Geometry check sheet. Reference: the model listing, model coordinates, mm. A direction names the side the tool comes from. Coordinates: 2 decimals unless noted, no trailing zeros. Order: outer loops, then holes, each group sorted by start corner. A loop starts at its lowest first (then second) coordinate and runs counter-clockwise, first axis right, second up.
```python
from build123d import *

# Parameters (mm, degrees)
SKETCH1_W     = 3.175
SKETCH1_H     = 12.7
CHAMFER1_SIZE = 1.27


with BuildPart() as part:
    # Sketch1 → Revolve1 (revolve)
    with BuildSketch(Plane.XY, mode=Mode.PRIVATE) as revolve1_sk:
        with BuildLine():
            ThreePointArc((-3.367596045, 31.557403955), (-1.822529847, 30.525023726), (0, 30.1625))
            Line((0, 30.1625), (0, 39.6875))
            ThreePointArc((0, 39.6875), (-3.367596045, 38.292596045), (-4.7625, 34.925))
            ThreePointArc((-4.7625, 34.925), (-4.670989898, 33.995882341), (-4.399976274, 33.102470153))
            ThreePointArc((-4.399976274, 33.102470153), (-3.959874029, 32.279096765), (-3.367596045, 31.557403955))
        make_face()
        with BuildLine():
            Line((-4.7625, 9.525), (0, 9.525))
            Line((0, 9.525), (0, 30.1625))
            ThreePointArc((0, 30.1625), (-1.822529847, 30.525023726), (-3.367596045, 31.557403955))
            ThreePointArc((-3.367596045, 31.557403955), (-3.959874029, 32.279096765), (-4.399976274, 33.102470153))
            ThreePointArc((-4.399976274, 33.102470153), (-2.411195624, 21.280368821), (-4.7625, 9.525))
        make_face()
        Polygon((-6.35, 6.35), (-3.175, 6.35), (0, 6.35), (0, 9.525), (-4.7625, 9.525), (-6.35, 9.525), align=None)
        with Locations((-1.5875, 0)):
            Rectangle(SKETCH1_W, SKETCH1_H)
    revolve(revolve1_sk.sketch.rotate(Axis((0, 45.924305238, 0), (0, 1, 0)), 180), axis=Axis((0, 45.924305238, 0), (0, 1, 0)))

    # Chamfer1
    chamfer1_edges = [part.edges().sort_by_distance(p)[0] for p in [
        (-6.35, 9.525, 0),
    ]]
    chamfer(chamfer1_edges, length=CHAMFER1_SIZE)


solid = part.part
```
Item 1: Sectioned sample at C-C (y = 23.5). Record the cut outline in (x, z).
Item 2: Tool access check on faces 1 (the face through (0, -6.35, 0)), 2 (the face through (1.5, 0.1, 2.8)). Record the directions out of +Z, -Z, +X, -X, +Y, -Y that give a thin tool (end or side, any length) a straight path to the whole face; none if there is none.
Item 3: Thickness scan on line 1 along Y through (x, z) = (-2.5, -3.5); line 2 along Y through (x, z) = (1.5, 5); line 3 along X through (y, z) = (5, -0.5). Record the ranges inside material, lowest first.
Item 4: Sectioned sample at D-D (y = 9). Record the cut outline in (x, z) (3 decimals), and give its area (3 significant figures).
Item 5: Depth check by flat-ended pin: P1, Ø5, axis at x = -2.5, y = 27, coming from the +Z side; P2, Ø1.5, axis at y = 0, z = -2.5, coming from the +X side; P3, Ø3, axis at x = -2.5, y = 4.5, coming from the +Z side. Enter the tip coordinate at first touch or a pass-through.
Geometry check:
1. outline: circle Ø4.9 at (0, 0)
2. face 1: +Z, -Z, +X, -X, -Y
2. face 2: -Y
3. line 1: y = 6.35 to 10.75, 32.83 to 36.97
3. line 2: y = 6.35 to 9.38
3. line 3: x = -3.14 to 3.14
4. outline: circle Ø11.21 at (0, 0)
4. area: 98.7 mm2
5. P1: stops at z = 3.07
5. P2: stops at x = 2.65
5. P3: stops at z = 3.01
